Answer from the drawing. Dimensions are ordinates in mm from the lowest x, y and z of the part. Give positions to 0.01 mm unless a question says otherwise; leave off trailing zeros. Order: outer loops, then holes, each group sorted by start corner. A loop starts at its lowest first (then second) coordinate and runs counter-clockwise, first axis right, second up.
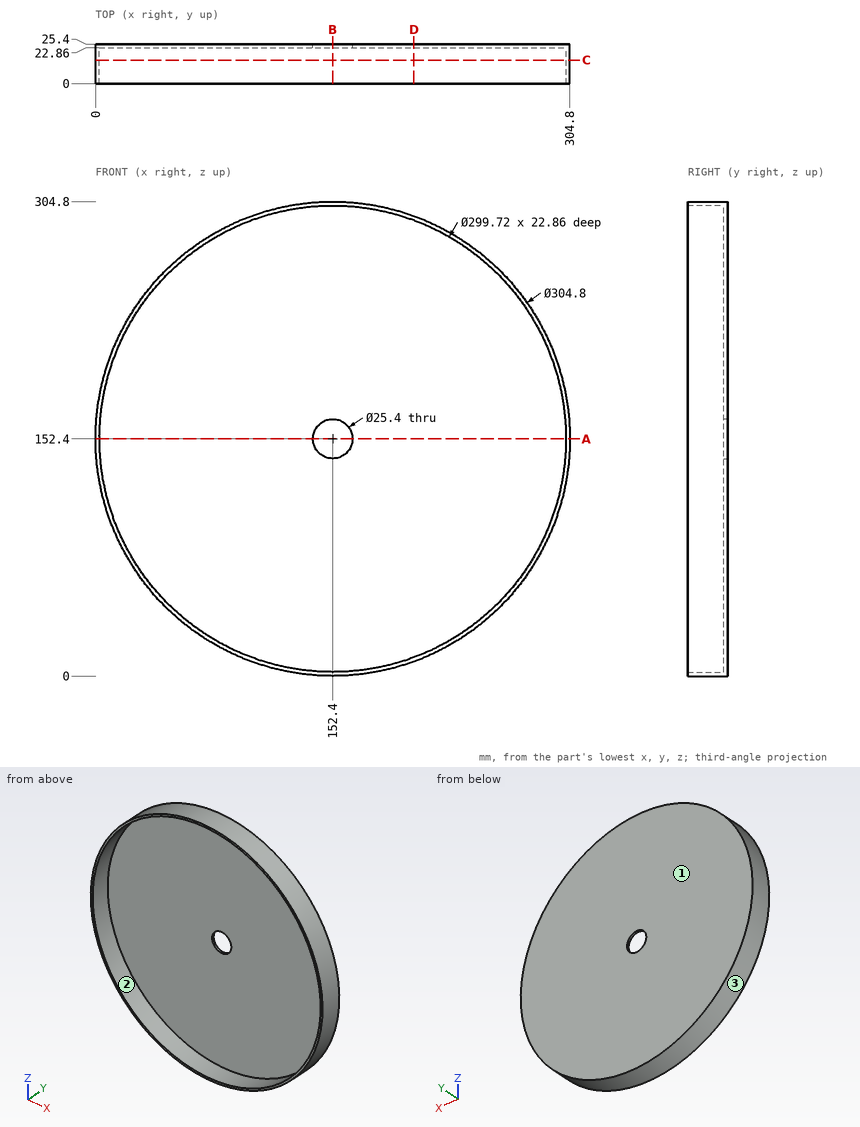
1. The mould has two halves that part along Z. Classify the marked faces 1, 2 and 3: pulls with the +Z half, pulls with the -Z half, needs draft (parallel to the pull), parting line crosses it, or undercut.
Findings below:
face 1: needs draft
face 2: undercut
face 3: parting line crosses it
2. The part is cut by section A-A (z = 152.4). Write down the section's boundary in (x, y), then the cut area to 3 significant figures.
Findings below:
outline: (0, 0) - (2.54, 0) - (2.54, 22.86) - (139.7, 22.86) - (139.7, 25.4) - (0, 25.4) - close; (165.1, 22.86) - (302.26, 22.86) - (302.26, 0) - (304.8, 0) - (304.8, 25.4) - (165.1, 25.4) - close
area: 826 mm2
3. Straight lines are drawn through the part: probe 1 along X at (y, z) = (13.5, 152.4); probe 2 along Y at (x, z) = (50, 68); probe 3 along Z at (x, y) = (180.5, 23). For each, find the intervals that lie inside material, in ascending order.
Findings below:
probe 1: x = 0 to 2.54, 302.26 to 304.8
probe 2: y = 22.86 to 25.4
probe 3: z = 2.61 to 302.19
4. The part is cut by section B-B (x = 152.4). Write down the section's boundary in (y, z).
Findings below:
outline: (0, 0) - (25.4, 0) - (25.4, 139.7) - (22.86, 139.7) - (22.86, 2.54) - (0, 2.54) - close; (0, 302.26) - (22.86, 302.26) - (22.86, 165.1) - (25.4, 165.1) - (25.4, 304.8) - (0, 304.8) - close
5. The part is cut by section D-D (x = 204.5). Write down the section's boundary in (y, z), then the cut area to 3 significant figures.
Findings below:
outline: (0, 9.18) - (25.4, 9.18) - (25.4, 295.62) - (0, 295.62) - (0, 292.91) - (22.86, 292.91) - (22.86, 11.89) - (0, 11.89) - close
area: 851 mm2
6. Given P1, Ø6, axis at x = 167.5, y = 5, coming from the +Z side; P2, Ø20.5, axis at x = 152.4, z = 152.4, coming from the -Y side; P3, Ø3, axis at y = 11.5, z = 267, coming from the -X side; P4, Ø8, axis at y = 21.5, z = 204.5, coming from the +X side, each flat-ended and moving along its own axis, determine where each tip first touches the part or whether it passes through.
Findings below:
P1: stops at z = 304.32
P2: passes through
P3: stops at x = 50.25
P4: stops at x = 297.01
7. The part is cut by section C-C (y = 15). Write down the section's boundary in (x, z).
Findings below:
outline: circle Ø304.8 at (152.4, 152.4); hole circle Ø299.72 at (152.4, 152.4)
